Design review of the part built by this model. Coordinates are the model's own, in mm. Give positions to 0.01 mm unless a question says otherwise; leave off trailing zeros. Order: outer loops, then holes, each group sorted by start corner. A loop starts at its lowest first (then second) coordinate and runs counter-clockwise, first axis right, second up. Notation, with made-up numbers: (75.25, -16) -> (116.25, -16) arc R11 ccw to (116.25, 0) -> close; hole circle Ø9 at (-32, -39.5). An arc over 180 degrees is marked (long way). Return JSON: item names as keys, results as strings.
```python
from build123d import *

# Parameters (mm, degrees)
BOSS_EXTRUDE1_DEPTH = 25
SKETCH2_OUTSIDE_W   = 153.338
SKETCH2_OUTSIDE_H   = 142.664
SKETCH2_OUTSIDE_R   = 34.5
CUT_EXTRUDE1_DEPTH  = 25
CUT_EXTRUDE1_TAPER  = 45
SKETCH3_R           = 18.5
CUT_EXTRUDE2_DEPTH  = 26


with BuildPart() as part:
    # Sketch1 → Boss-Extrude1 (new body)
    with BuildSketch(Plane(origin=(0, 0, 0), x_dir=(1, 0, 0), z_dir=(0, 1, 0))):
        Polygon((19.918584287, 34.5), (-19.918584287, 34.5), (-39.837168574, 0), (-19.918584287, -34.5), (19.918584287, -34.5), (39.837168574, 0), align=None)
    extrude(amount=BOSS_EXTRUDE1_DEPTH)

    # Sketch2 outside → Cut-Extrude1 (cut)
    with BuildSketch(Plane(origin=(0, 25, 0), x_dir=(1, 0, 0), z_dir=(0, 1, 0))):
        Rectangle(SKETCH2_OUTSIDE_W, SKETCH2_OUTSIDE_H)
        Circle(SKETCH2_OUTSIDE_R, mode=Mode.SUBTRACT)
    extrude(amount=-CUT_EXTRUDE1_DEPTH, taper=CUT_EXTRUDE1_TAPER, mode=Mode.SUBTRACT)

    # Sketch3 → Cut-Extrude2 (cut, through all)
    with BuildSketch(Plane(origin=(0, 25, 0), x_dir=(1, 0, 0), z_dir=(0, 1, 0))):
        Circle(SKETCH3_R)
    extrude(amount=-CUT_EXTRUDE2_DEPTH, mode=Mode.SUBTRACT)


solid = part.part
```
Item 1: Add section A-A (y = 5). Give the boundary of the cut face in (x, z).
Result set:
{"outline": "(-39.84, 0) -> (-19.92, -34.5) -> (19.92, -34.5) -> (39.84, 0) -> (19.92, 34.5) -> (-19.92, 34.5) -> close; hole circle Ø37 at (0, 0)"}
Item 2: Mouldability with a two-part tool opening along X and no side actions: class faces 1 (the face through (29.74, 12.33, 17.49)), 2 (the face through (-35.8, 23.7, 0.1)), 3 (the face through (-4.01, 12.68, 18.06)) as released by +X, released by -X, zero draft, split by the parting line, or undercut.
Result set:
{"face 1": "released by +X", "face 2": "released by -X", "face 3": "undercut"}
Item 3: For pin 1 (6 mm diameter, centred on x = 26.5, y = 6.5, fed in from -Z); pin 2 (3 mm diameter, centred on x = 29.5, y = 6, fed in from +Z); pin 3 (3 mm diameter, centred on x = -31.5, y = 14, fed in from +Z), all flat-tipped, find the tip position at first contact; note any pin that passes through.
Result set:
{"pin 1": "stops at z = -28.3", "pin 2": "stops at z = 20.5", "pin 3": "stops at z = 17.04"}
Item 4: Wall thickness on L1, parallel to X at y = 8.75, z = 0; L2, parallel to Z at x = 0, y = 15.25; L3, parallel to Z at x = 11.5, y = 20.75: over which ranges is each line inside the solid? List them lowest first. Write a range as [from, to].
Result set:
{"L1": "x = [-39.84, -18.5], [18.5, 39.84]", "L2": "z = [-34.5, -18.5], [18.5, 34.5]", "L3": "z = [-34.5, -14.49], [14.49, 34.5]"}
